from build123d import *

# Parameters (mm, degrees)
F0_W = 4
F0_H = 4
F2_R = 0.99999


# Not quite as in the source:
# - a fillet or chamfer is up to 0.001 mm smaller than in the source, because OpenCascade refuses the exact size
# - the dataset's text gives a spline's control points without its knots; the knots are read off the source's solid


with BuildPart() as f1:
    # F0 (on Front) → F1 (revolve)
    with BuildSketch(Plane.XZ):
        with BuildLine():
            Line((0.9091711268, 3), (-3.0908288732, 3))
            add(Edge.make_bspline(
                [(-3.0908288732, 3), (-3.5834098611, 2.4200538723), (-4.8095609066, 0.976430248), (-8.1139250982, 0.3655009849), (-10.0908288732, 0)],
                knots=[0, 0, 0, 0, 0.4017294522, 1, 1, 1, 1], degree=3))
            Line((-10.0908288732, 0), (-9.7272200714, -1.9666694281))
            add(Edge.make_bspline(
                [(-1.5664662541, 1.7052727679), (-1.7197351348, 1.5248198149), (-2.063357916, 1.1180932901), (-2.6429158857, 0.5377987308), (-3.2231154482, 0.0813793664), (-3.7171330132, -0.2427740222), (-4.2708452388, -0.5352938299), (-4.8332722817, -0.7761481117), (-5.411616192, -0.9839057168), (-6.200976021, -1.2257159643), (-7.2204637167, -1.4786072566), (-8.4760577728, -1.735410051), (-9.3141745474, -1.8903032702), (-9.7272200714, -1.9666694281)],
                knots=[0, 0, 0, 0, 0.125, 0.25, 0.3125, 0.375, 0.4375, 0.5, 0.5625, 0.625, 0.75, 0.875, 1, 1, 1, 1], degree=3))
            Line((-1.5664662541, 1.7052727679), (0.9091711268, 3))
        make_face()
        with Locations((-1.0908288732, 5)):
            Rectangle(F0_W, F0_H)
    revolve(axis=Axis((0.9091711268, 0, 5), (0, 0, 1)))

    # F2 (radius 1 in the source; OpenCascade refuses exactly that, so slightly less here)
    f2_edges = [f1.edges().sort_by_distance(p)[0] for p in [
        (11.545562, 0, -1.966669),
        (11.909171, 0, 0),
    ]]
    fillet(f2_edges, radius=F2_R)


solid = f1.part
Model file for the job. Use its own axes, mm. Coordinates: 2 decimals unless noted, no trailing zeros. Order: outer loops, then holes, each group sorted by start corner. A loop starts at its lowest first (then second) coordinate and runs counter-clockwise, first axis right, second up. Notation, with made-up numbers: (56.25, -22.5) -> (101.25, -22.5) arc R17 cw to (101.25, -15.5) -> close; hole circle Ø11 at (-6, 59.5). An arc over 180 degrees is marked (long way). Return JSON: item names as keys, results as strings. Group by question number.
Item 1: Flat gauge pins, fed straight in: P1, Ø1, axis at x = 8.5, y = 3.5, coming from the -Z side; P2, Ø4, axis at x = 1, y = 4, coming from the -Z side; P3, Ø5, axis at x = -4, z = 2.5, coming from the -Y side; P4, Ø2, axis at x = 0, z = -0.5, coming from the +Y side. Where does each tip first touch, or does it go through?
Item 2: Pull direction X, two halves, no side cores. Call faces 1 (the conical face through (1.223, 0.241, 2.793)), 2 (the flat face through (1, 0, 7)), 3 (the cylindrical face through (1.8, 3.9, 5)): pulls with the +X half, pulls with the -X half, needs draft (parallel to the pull), parting line crosses it, or undercut.
Item 3: Wall check: line 1 along X through (y, z) = (2.25, -0.25); line 2 along Y through (x, z) = (3, 1.25); line 3 along X through (y, z) = (0.5, 4). Give the ranges that are in metal, low to high. Write a range as [from, to].
Item 4: Saw through at A-A on z = 5.5. Write the cut outline in (x, y), then the cut area to 3 significant figures.
Values found:
{
 "1": {"P1": "stops at z = -1.63", "P2": "stops at z = -0.87", "P3": "stops at y = -9.38", "P4": "stops at y = 10.84"},
 "2": {"face 1": "undercut", "face 2": "needs draft", "face 3": "parting line crosses it"},
 "3": {"line 1": "x = [-9.52, -3.17], [4.99, 11.34]", "line 2": "y = [-5.73, -1.97], [1.97, 5.73]", "line 3": "x = [-3.06, 4.88]"},
 "4": {"outline": "circle Ø8 at (0.91, 0)", "area": "50.3 mm2"}
}
